Check sheet for the modelled part. Datum: model origin and axes. Units: mm. A direction names the side the tool comes from. Round coordinates to 2 decimals unless told otherwise and drop trailing zeros. Write each loop counter-clockwise with the first axis right and the second up, starting at its lowest first coordinate (ties: lowest second). Pieces come first, ordered by that corner, then holes. Notation, with made-up numbers: M 29,-40 L 87,-40 A21 cw 87,-33 Z; hole C 17,37.25 d10. An arc over 180 degrees is marked long. One line per item, written item: value.
from build123d import *

# Parameters (mm, degrees)
F1_DEPTH = 3
F3_D     = 3.7973
F4_W     = 1.27
F4_H     = 44.4500002354
F4_H_2   = 44.45
F5_DEPTH = 3.001
F6_R     = 0.63499


# Not quite as in the source:
# - a fillet or chamfer is up to 0.001 mm smaller than in the source, because OpenCascade refuses the exact size


with BuildPart() as f1:
    # F0 (on Front) → F1 (new body)
    with BuildSketch(Plane.XZ):
        Polygon((38.1, 25.4), (-38.1, 25.4), (-38.1, 12.7), (-35.1, 12.7), (-35.1, 6.35), (-38.1, 6.35), (-38.1, -6.35), (-35.1, -6.35), (-35.1, -12.7), (-38.1, -12.7), (-38.1, -25.4), (-31.75, -25.4), (-31.75, -22.4), (-27.1526, -22.4), (-27.1526, -18.6436), (-29.3624, -18.6436), (-29.3624, -15.875), (-27.1526, -15.875), (-27.1526, -12.7), (-23.6474, -12.7), (-23.6474, -15.875), (-21.4376, -15.875), (-21.4376, -18.6436), (-23.6474, -18.6436), (-23.6474, -22.4), (-19.05, -22.4), (-19.05, -25.4), (38.1, -25.4), align=None)
    extrude(amount=F1_DEPTH)

    # F3 (through all)
    with Locations(Plane.XZ.offset(3)):
        with Locations((-36.6, 0)):
            Hole(F3_D / 2)

    # F4 (on face) → F5 (cut, through all)
    with BuildSketch(Plane.XZ.offset(3)):
        with Locations((-6.3499999233, 3.1749998823)):
            Rectangle(F4_W, F4_H)
        with Locations((-2.5399999233, -3.175)):
            Rectangle(F4_W, F4_H_2)
        with Locations((5.0800000767, -3.175)):
            Rectangle(F4_W, F4_H_2)
        with Locations((1.2700000767, 3.1749998823)):
            Rectangle(F4_W, F4_H)
        with Locations((12.7000000767, -3.175)):
            Rectangle(F4_W, F4_H_2)
        with Locations((8.8900000767, 3.1749998823)):
            Rectangle(F4_W, F4_H)
        with Locations((20.3200000767, -3.175)):
            Rectangle(F4_W, F4_H_2)
        with Locations((16.5100000767, 3.1749998823)):
            Rectangle(F4_W, F4_H)
        with Locations((27.9400000767, -3.175)):
            Rectangle(F4_W, F4_H_2)
        with Locations((24.1300000767, 3.1749998823)):
            Rectangle(F4_W, F4_H)
    extrude(amount=-F5_DEPTH, mode=Mode.SUBTRACT)

    # F6 (radius 0.635 in the source; OpenCascade refuses exactly that, so slightly less here)
    f6_edges = [f1.edges().sort_by_distance(p)[0] for p in [
        (-6.985, -1.5, -19.05),
        (-5.715, -1.5, -19.05),
        (0.635, -1.5, -19.05),
        (1.905, -1.5, -19.05),
        (9.525, -1.5, -19.05),
        (8.255, -1.5, -19.05),
        (15.875, -1.5, -19.05),
        (17.145, -1.5, -19.05),
        (24.765, -1.5, -19.05),
        (23.495, -1.5, -19.05),
        (-3.175, -1.5, 19.05),
        (4.445, -1.5, 19.05),
        (12.065, -1.5, 19.05),
        (19.685, -1.5, 19.05),
        (27.305, -1.5, 19.05),
        (-1.905, -1.5, 19.05),
        (5.715, -1.5, 19.05),
        (13.335, -1.5, 19.05),
        (20.955, -1.5, 19.05),
        (28.575, -1.5, 19.05),
        (-1.905, -1.5, -25.4),
        (4.445, -1.5, -25.4),
        (5.715, -1.5, -25.4),
        (12.065, -1.5, -25.4),
        (13.335, -1.5, -25.4),
        (19.685, -1.5, -25.4),
        (20.955, -1.5, -25.4),
        (27.305, -1.5, -25.4),
        (28.575, -1.5, -25.4),
        (-6.985, -1.5, 25.4),
        (-5.715, -1.5, 25.4),
        (-3.175, -1.5, -25.4),
        (0.635, -1.5, 25.4),
        (1.905, -1.5, 25.4),
        (8.255, -1.5, 25.4),
        (9.525, -1.5, 25.4),
        (15.875, -1.5, 25.4),
        (17.145, -1.5, 25.4),
        (23.495, -1.5, 25.4),
        (24.765, -1.5, 25.4),
    ]]
    fillet(f6_edges, radius=F6_R)


solid = f1.part
Q1. Scan lines: line 1 (X direction, y = -1.85, z = 22.5) (3 decimals); line 2 (Z direction, x = -36.6, y = -1.6); line 3 (Z direction, x = 20, y = -2.8). Record each from-to range of solid material in increasing order. Write a range as [from, to].
Completed:
line 1: [-38.1, -6.985], [-5.715, 0.635], [1.905, 8.255], [9.525, 15.875], [17.145, 23.495], [24.765, 38.1]
line 2: [-25.4, -12.7], [-6.35, -1.9], [1.9, 6.35], [12.7, 25.4]
line 3: [18.96, 25.4]
Q2. Access from +Z, -Z, +X, -X, +Y, -Y to the whole of each face (thin tool, end or side, straight path). Record for faces 4 (the flat face through (-29, -1, -22.4)), 5 (the flat face through (-5.715, -2, 3)), 6 (the flat face through (32, -1, 25.4)), 7 (the flat face through (-35.1, -1, 10)).
Completed:
face 4: -Z, +Y, -Y
face 5: +Z, +Y, -Y
face 6: +Z, +X, -X, +Y, -Y
face 7: -X, +Y, -Y
Q3. Sectioned sample at B-B on z = 5. State how many separate pieces and enclosed holes the cut face has, and give its area (4 significant figures).
Completed:
separate pieces: 11
enclosed holes: 0
area: 190.5 mm^2
Q4. Depth check by flat-ended pin: P1, Ø1.5, axis at x = -25.5, y = -2, coming from the -Z side; P2, Ø1.5, axis at y = -1.5, z = -10, coming from the -X side; P3, Ø12, axis at x = 19, z = 12.5, coming from the +Y side. Enter the tip coordinate at first touch or a pass-through.
Completed:
P1: z = -12.7
P2: x = -35.1
P3: y = 0
Q5. Draft check along Z on faces 1 (the flat face through (-1, -3, 0)), 2 (the flat face through (5, -1, 25.4)), 3 (the flat face through (-35.1, -1, -9)). Enter one of: pulls with the +Z half, pulls with the -Z half, needs draft (parallel to the pull), parting line crosses it, or undercut.
Completed:
face 1: needs draft
face 2: pulls with the +Z half
face 3: undercut
Q6. Sectioned sample at A-A on x = -36.6. Enter the section's corners in (y, z), and give its area (3 significant figures).
Completed:
outline: M -3,-25.4 L 0,-25.4 L 0,-12.7 L -3,-12.7 Z; M -3,-6.35 L 0,-6.35 L 0,-1.9 L -3,-1.9 Z; M -3,1.9 L 0,1.9 L 0,6.35 L -3,6.35 Z; M -3,12.7 L 0,12.7 L 0,25.4 L -3,25.4 Z
area: 103 mm^2
